Input: part model. Units: mm. Frame: model coordinates. Face numbers are marked on the shaded views. A direction names the side the tool comes from. Round coordinates to 2 decimals unless told otherwise and drop trailing zeros. Loops run counter-clockwise (first coordinate to the right, second up) from the corner with the lowest first, then second, coordinate; pieces in that order, holes last. Notation, with made-up numbers: (-28, 14) -> (16, 14) arc R25 ccw to (16, 48) -> close; hole circle Ø1 at (-21.5, -36.75). An arc over 180 degrees is marked (long way). Answer as a JSON object with one key per item and string values.
```python
from build123d import *

# Parameters (mm, degrees)
SKETCH1_W           = 160
SKETCH1_H           = 30
BOSS_EXTRUDE1_DEPTH = 80
SHELL1_T            = -5
SKETCH2_R           = 4.17592015
CUT_EXTRUDE1_DEPTH  = 15
LPATTERN1_COUNT     = 4
LPATTERN1_PITCH     = 110


with BuildPart() as part:
    # Sketch1 → Boss-Extrude1 (new body)
    with BuildSketch(Plane.XY):
        with Locations((34.869684499, 8.141289438)):
            Rectangle(SKETCH1_W, SKETCH1_H)
    extrude(amount=BOSS_EXTRUDE1_DEPTH)

    # Shell1
    shell1_openings = [part.faces().sort_by_distance(p)[0] for p in [
        (34.869684499, -6.858710562, 40),
    ]]
    offset(amount=SHELL1_T, openings=shell1_openings, kind=Kind.INTERSECTION)

    # Sketch2 → Cut-Extrude1 (cut)
    with BuildSketch(Plane(origin=(0, 0, 0), x_dir=(-1, 0, 0), z_dir=(0, 0, -1))):
        with Locations((30.130315501, 7.814471991)):
            Circle(SKETCH2_R)
    cut_extrude1 = extrude(amount=-CUT_EXTRUDE1_DEPTH, mode=Mode.SUBTRACT)

    # LPattern1: Cut-Extrude1 ×4
    with Locations(*[(i * LPATTERN1_PITCH, 0, 0) for i in range(1, LPATTERN1_COUNT)]):
        add(cut_extrude1, mode=Mode.SUBTRACT)


solid = part.part
```
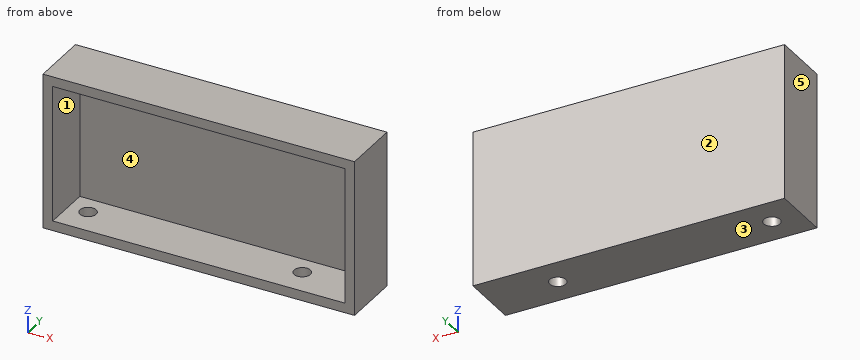
1) Ray query, probe 1 along Z at (x, y) = (49, 4.25); probe 2 along X at (y, z) = (6.75, 71); probe 3 along Y at (x, z) = (70.5, 27). Return the intervals inside material, ascending.
Output:
{"probe 1": "z = 0 to 5, 75 to 80", "probe 2": "x = -45.13 to -40.13, 109.87 to 114.87", "probe 3": "y = 18.14 to 23.14"}
2) Section B-B, the plane z = 72. Output: boundary loops of the cut face in (x, y), plus the area to 3 significant figures.
Output:
{"outline": "(-45.13, -6.86) -> (-40.13, -6.86) -> (-40.13, 18.14) -> (109.87, 18.14) -> (109.87, -6.86) -> (114.87, -6.86) -> (114.87, 23.14) -> (-45.13, 23.14) -> close", "area": "1,050 mm^2"}
3) Section A-A, the plane x = -31. Output: boundary loops of the cut face in (y, z).
Output:
{"outline": "(-6.86, 0) -> (3.73, 0) -> (3.73, 5) -> (-6.86, 5) -> close; (-6.86, 75) -> (18.14, 75) -> (18.14, 5) -> (11.9, 5) -> (11.9, 0) -> (23.14, 0) -> (23.14, 80) -> (-6.86, 80) -> close"}
4) Reachability of the marked faces 1 and 2 from +Z, -Z, +X, -X, +Y, -Y: full face, straight path, thin tool, end or side. Return the list, or none.
Output:
{"face 1": "-Y", "face 2": "+Z, -Z, +X, -X, +Y"}
5) Draft query along X for the marked faces 3, 4 and 5. Return one class per face: +X half, -X half, draft (parallel to the pull), parting line (faces both ways), or undercut.
Output:
{"face 3": "draft", "face 4": "undercut", "face 5": "-X half"}
6) Section C-C, the plane x = 73. Output: boundary loops of the cut face in (y, z).
Output:
{"outline": "(-6.86, 0) -> (23.14, 0) -> (23.14, 80) -> (-6.86, 80) -> (-6.86, 75) -> (18.14, 75) -> (18.14, 5) -> (-6.86, 5) -> close"}
